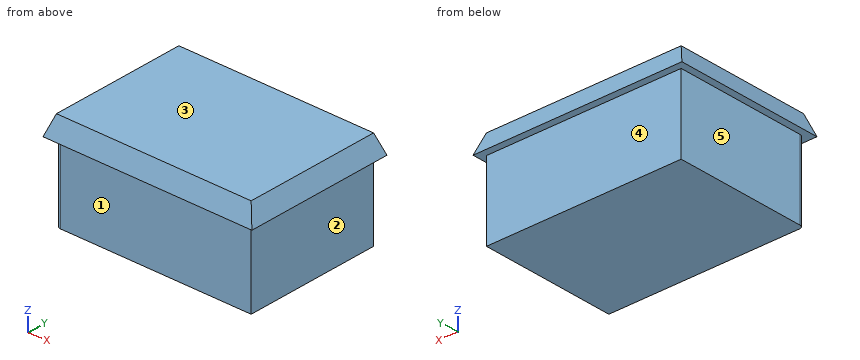
from build123d import *

# Parameters (mm, degrees)
F0_W      = 254
F0_H      = 177.8
F1_DEPTH  = 127
F1_FACE_W = 254
F1_FACE_H = 177.8
F2_DEPTH  = 25.4
F2_TAPER  = -20
F3_R      = 5.08


with BuildPart() as f1:
    # F0 (on Top) → F1 (new body)
    with BuildSketch(Plane.XY):
        Rectangle(F0_W, F0_H)
    extrude(amount=F1_DEPTH)

    # F1_face (on face) → F2 (join)
    with BuildSketch(Plane.XY.offset(127)):
        Rectangle(F1_FACE_W, F1_FACE_H)
    extrude(amount=-F2_DEPTH, taper=F2_TAPER)

    # F3
    f3_edges = [f1.edges().sort_by_distance(p)[0] for p in [
        (-127, -88.9, 50.8),
    ]]
    fillet(f3_edges, radius=F3_R)


solid = f1.part
Source: CAD feature listing. Evaluate the final solid. Frame: model axes, mm. Face numbers are marked on the shaded views. A direction names the side the tool comes from. Round coordinates to 2 decimals unless told otherwise and drop trailing zeros. Loops run counter-clockwise (first coordinate to the right, second up) from the corner with the lowest first, then second, coordinate; pieces in that order, holes last. Notation, with made-up numbers: (54.5, 60.5) - (78.5, 60.5) arc R24 ccw to (78.5, 93.5) - close; hole circle Ø3 at (78.5, 36). An arc over 180 degrees is marked (long way). Write item = value, one per line. Start each with the question number.
Item 1: Section query A-A on z = 26.5. Output: boundary loops of the cut face in (x, y).
Item 2: Reachability of the marked faces 1, 2, 3, 4 and 5 from +Z, -Z, +X, -X, +Y, -Y: full face, straight path, thin tool, end or side. Return the list, or none.
Item 3: First-contact query: pin 1 Ø12 at (x, z) = (89.5, 41) entering from -Y; pin 2 Ø6 at (y, z) = (73.5, 18) entering from -X; pin 3 Ø10 at (x, z) = (-99.5, 49) entering from +Y. Flat tips, straight axial feed; report the tip coordinate or a pass-through.
Item 4: Material intervals for line 1 (X direction, y = -26, z = 51); line 2 (Y direction, x = -112.5, z = 33); line 3 (Y direction, x = -94, z = 113), sorted ascending.
Results list:
q1.outline = (-127, -83.82) arc R5.08 ccw to (-121.92, -88.9) - (127, -88.9) - (127, 88.9) - (-127, 88.9) - close
q2.face_1 = -Z, +X, -X, -Y
q2.face_2 = -Z, +X, +Y, -Y
q2.face_3 = +Z, +X, -X, +Y, -Y
q2.face_4 = -Z, +X, -X, +Y
q2.face_5 = -Z, -X, +Y, -Y
q3.pin_1 = -88.9
q3.pin_2 = -127
q3.pin_3 = 88.9
q4.line_1 = -127 to 127
q4.line_2 = -88.9 to 88.9
q4.line_3 = -94 to 94
